Work out the finished part from the listing and answer in its coordinate system (mm). A direction names the side the tool comes from. Give positions to 0.01 mm unless a question says otherwise; leave off trailing zeros. Loops run counter-clockwise (first coordinate to the right, second up) from the corner with the lowest first, then second, coordinate; pieces in that order, holes last. Notation, with made-up numbers: M 33.25,-24.75 L 63.25,-24.75 A34 cw 63.25,13.25 Z; hole C 13.5,73.25 d7. An arc over 180 degrees is marked long. Answer in a Markdown table with one row per item. Add a question column.
from build123d import *

# Parameters (mm, degrees)
SKETCH1_W           = 203.2
SKETCH1_H           = 88.9
SKETCH1_R           = 25.4
SKETCH1_R_2         = 4.064
BOSS_EXTRUDE1_DEPTH = 12.7
FILLET1_R           = 6.35


with BuildPart() as part:
    # Sketch1 → Boss-Extrude1 (new body)
    with BuildSketch(Plane(origin=(0, 0, 0), x_dir=(1, 0, 0), z_dir=(0, 1, 0))):
        with Locations((101.6, 44.45)):
            Rectangle(SKETCH1_W, SKETCH1_H)
        with Locations(Location((101.6, 44.45, 0), (0, 0, 270))):
            Circle(SKETCH1_R, mode=Mode.SUBTRACT)
        with Locations(Location((19.05, 19.05, 0), (0, 0, 270))):
            Circle(SKETCH1_R_2, mode=Mode.SUBTRACT)
        with Locations(Location((19.05, 44.45, 0), (0, 0, 270))):
            Circle(SKETCH1_R_2, mode=Mode.SUBTRACT)
        with Locations(Location((19.05, 69.85, 0), (0, 0, 270))):
            Circle(SKETCH1_R_2, mode=Mode.SUBTRACT)
        with Locations(Location((184.15, 69.85, 0), (0, 0, 90))):
            Circle(SKETCH1_R_2, mode=Mode.SUBTRACT)
        with Locations(Location((184.15, 44.45, 0), (0, 0, 90))):
            Circle(SKETCH1_R_2, mode=Mode.SUBTRACT)
        with Locations(Location((184.15, 19.05, 0), (0, 0, 90))):
            Circle(SKETCH1_R_2, mode=Mode.SUBTRACT)
        with BuildLine():
            Line((38.1, 73.914), (69.85, 73.914))
            ThreePointArc((69.85, 73.914), (73.914, 69.85), (69.85, 65.786))
            Line((69.85, 65.786), (38.1, 65.786))
            ThreePointArc((38.1, 65.786), (34.036, 69.85), (38.1, 73.914))
        make_face(mode=Mode.SUBTRACT)
        with BuildLine():
            Line((38.1, 14.986), (69.85, 14.986))
            ThreePointArc((69.85, 14.986), (73.914, 19.05), (69.85, 23.114))
            Line((69.85, 23.114), (38.1, 23.114))
            ThreePointArc((38.1, 23.114), (34.036, 19.05), (38.1, 14.986))
        make_face(mode=Mode.SUBTRACT)
        with BuildLine():
            Line((165.1, 14.986), (133.35, 14.986))
            ThreePointArc((133.35, 14.986), (129.286, 19.05), (133.35, 23.114))
            Line((133.35, 23.114), (165.1, 23.114))
            ThreePointArc((165.1, 23.114), (169.164, 19.05), (165.1, 14.986))
        make_face(mode=Mode.SUBTRACT)
        with BuildLine():
            Line((165.1, 73.914), (133.35, 73.914))
            ThreePointArc((133.35, 73.914), (129.286, 69.85), (133.35, 65.786))
            Line((133.35, 65.786), (165.1, 65.786))
            ThreePointArc((165.1, 65.786), (169.164, 69.85), (165.1, 73.914))
        make_face(mode=Mode.SUBTRACT)
    extrude(amount=BOSS_EXTRUDE1_DEPTH)

    # Fillet1
    fillet1_edges = [part.edges().sort_by_distance(p)[0] for p in [
        (0, 6.35, -88.9),
        (203.2, 6.35, -88.9),
        (203.2, 6.35, 0),
        (0, 6.35, 0),
    ]]
    fillet(fillet1_edges, radius=FILLET1_R)


solid = part.part
(1) This flat-tipped pin is pushed along its axis until it touches: P1, Ø13, axis at x = 184.15, z = -19.05, coming from the +Y side. Where does it stop, or does it pass through?
(2) Which of the six approach directions +Z, -Z, +X, -X, +Y, -Y give full straight-line access (tool end or side, diameter ignored) to faces 1 (the face through (78, 12.7, -55)), 2 (the face through (34.037, 6.261, -19.139))?
(3) Section A-A, the plane x = 19.05 is taken. Determine the outline of the cut face in (y, z).
(4) The mould has two halves that part along Z. Classify faces 3 (the face through (149, 6, -65.786)), 4 (the face through (201.29, 6.44, -87.09)), 5 (the face through (203.2, 6, -44)), 6 (the face through (76.804, 6.261, -49.956)): pulls with the +Z half, pulls with the -Z half, needs draft (parallel to the pull), parting line crosses it, or undercut.
(5) Section B-B, the plane x = 156.5 is taken. Determine the outline of the cut face in (y, z), and give its area (3 significant figures).
(6) Consider line 1 along Z through (x, y) = (65.5, 5); line 2 along Z through (x, y) = (184.15, 9.75); line 3 along X through (y, z) = (4, -67). Determine where each line is inside the solid, lowest interval first. Write a range as from..to.
(7) Section C-C, the plane y = 3.25 is taken. State how many separate pieces and enclosed holes the cut face has, and give its area (3 significant figures).
(8) Section D-D, the plane z = -44.45 is taken. Determine the outline of the cut face in (x, y), and give its area (3 significant figures).
Numbers:
| question | item | result |
|---|---|---|
| 1 | P1 | stops at y = 12.7 |
| 2 | face 1 | +Z, -Z, +X, -X, +Y |
| 2 | face 2 | +Y, -Y |
| 3 | outline | M 0,-88.9 L 12.7,-88.9 L 12.7,-73.91 L 0,-73.91 Z; M 0,-65.79 L 12.7,-65.79 L 12.7,-48.51 L 0,-48.51 Z; M 0,-40.39 L 12.7,-40.39 L 12.7,-23.11 L 0,-23.11 Z; M 0,-14.99 L 12.7,-14.99 L 12.7,0 L 0,0 Z |
| 4 | face 3 | undercut |
| 4 | face 4 | pulls with the -Z half |
| 4 | face 5 | needs draft |
| 4 | face 6 | undercut |
| 5 | outline | M 0,-88.9 L 12.7,-88.9 L 12.7,-73.91 L 0,-73.91 Z; M 0,-65.79 L 12.7,-65.79 L 12.7,-23.11 L 0,-23.11 Z; M 0,-14.99 L 12.7,-14.99 L 12.7,0 L 0,0 Z |
| 5 | area | 923 mm² |
| 6 | line 1 | z = -88.9..-73.91, -65.79..-23.11, -14.99..0 |
| 6 | line 2 | z = -88.9..-73.91, -65.79..-48.51, -40.39..-23.11, -14.99..0 |
| 6 | line 3 | x = 0..16.15, 21.95..35.2, 72.75..89.91, 113.29..130.45, 168..181.25, 187.05..203.2 |
| 7 | separate pieces | 1 |
| 7 | enclosed holes | 11 |
| 7 | area | 14,500 mm² |
| 8 | outline | M 0,0 L 14.99,0 L 14.99,12.7 L 0,12.7 Z; M 23.11,0 L 76.2,0 L 76.2,12.7 L 23.11,12.7 Z; M 127,0 L 180.09,0 L 180.09,12.7 L 127,12.7 Z; M 188.21,0 L 203.2,0 L 203.2,12.7 L 188.21,12.7 Z |
| 8 | area | 1,730 mm² |
